```python
from build123d import *

# Parameters (mm, degrees)
SKETCH1_W               = 60
SKETCH1_H               = 30
BOSS_EXTRUDE1_DEPTH     = 3
FILLET2_R               = 2
SKETCH4_W               = 5
SKETCH4_H               = 20
BOSS_EXTRUDE2_DEPTH     = 25
FILLET3_R               = 10
CUT_EXTRUDE3_DEPTH      = 50.145193051
CUT_EXTRUDE3_DEPTH_BACK = 50.145193051
SKETCH5_R               = 2.75
CUT_EXTRUDE4_DEPTH      = 2.5
CHAMFER1_SIZE           = 5


with BuildPart() as part:
    # Sketch1 → Boss-Extrude1 (new body)
    with BuildSketch(Plane(origin=(0, 0, 0), x_dir=(1, 0, 0), z_dir=(0, 1, 0))):
        Rectangle(SKETCH1_W, SKETCH1_H)
    extrude(amount=BOSS_EXTRUDE1_DEPTH)

    # Fillet2
    fillet2_edges = [part.edges().sort_by_distance(p)[0] for p in [
        (-30, 1.5, -15),
        (30, 1.5, -15),
        (30, 1.5, 15),
        (-30, 1.5, 15),
    ]]
    fillet(fillet2_edges, radius=FILLET2_R)

    # Sketch4 → Boss-Extrude2 (add)
    with BuildSketch(Plane(origin=(0, 3, 0), x_dir=(1, 0, 0), z_dir=(0, 1, 0))):
        with Locations((-5, 0)):
            Rectangle(SKETCH4_W, SKETCH4_H)
        with Locations((5, 0)):
            Rectangle(SKETCH4_W, SKETCH4_H)
    extrude(amount=BOSS_EXTRUDE2_DEPTH)

    # Fillet3
    fillet3_edges = [part.edges().sort_by_distance(p)[0] for p in [
        (5, 28, 10),
        (5, 28, -10),
        (-5, 28, -10),
        (-5, 28, 10),
    ]]
    fillet(fillet3_edges, radius=FILLET3_R - 0.0001)  # a hair under: the kernel refuses the full size

    # Sketch5 → Cut-Extrude3 (cut, two sides: drawn at the far end of the back side and taken through both)
    with BuildSketch(Plane.ZY.offset(7.5).offset(-CUT_EXTRUDE3_DEPTH_BACK)):
        with Locations((0, 18)):
            Circle(SKETCH5_R)
    extrude(amount=CUT_EXTRUDE3_DEPTH + CUT_EXTRUDE3_DEPTH_BACK, mode=Mode.SUBTRACT)

    # Sketch6 → Cut-Extrude4 (cut)
    with BuildSketch(Plane(origin=(7.5, 0, 0), x_dir=(0, 0, -1), z_dir=(1, 0, 0))):
        Polygon((0, 13.236860279), (4.125, 15.61843014), (4.125, 20.38156986), (0, 22.763139721), (-4.125, 20.38156986), (-4.125, 15.61843014), align=None)
    extrude(amount=-CUT_EXTRUDE4_DEPTH, mode=Mode.SUBTRACT)

    # Chamfer1
    chamfer1_edges = [part.edges().sort_by_distance(p)[0] for p in [
        (-5, 3, -10),
        (-5, 3, 10),
        (5, 3, -10),
        (5, 3, 10),
    ]]
    chamfer(chamfer1_edges, length=CHAMFER1_SIZE - 0.0001)  # a hair under: the kernel refuses the full size


solid = part.part
```
Design review of the part built by this model. Coordinates are the model's own, in mm. A direction names the side the tool comes from. Round coordinates to 2 decimals unless told otherwise and drop trailing zeros. Write each loop counter-clockwise with the first axis right and the second up, starting at its lowest first coordinate (ties: lowest second). Pieces come first, ordered by that corner, then holes.
Item 1: For faces 4 (the flat face through (0, 3, 0)), 5 (the flat face through (5, 13, -10)), 6 (the flat face through (6.27, 21.59, 2.03)), 7 (the flat face through (-5, 13, 10)), list the 3-axis set-ups (+Z, -Z, +X, -X, +Y, -Y) from which the entire face can be reached by the end or side of a thin tool; tool diameter is ignored.
Item 2: We need section B-B on y = 10. Write out the cut boundary in (x, z), and give its area (3 significant figures).
Item 3: The part is to be moulded in two halves that separate along Y. For faces 1 (the flat face through (7.5, 13, 0)), 2 (the flat face through (5, 6, 12)), 3 (the flat face through (6.268, 14.444, 2.091)), say which applies: +Y half, -Y half, draft (parallel to the pull), parting line (faces both ways), or undercut.
Item 4: We need section C-C on z = -2. Write out the cut boundary in (x, y).
Item 5: Clearance check with flat-ended pins moving along their axes: pin 1 Ø1.5 at (y, z) = (4, 0.5) entering from +X; pin 2 Ø10 at (y, z) = (21.5, -1) entering from -X; pin 3 Ø4 at (x, y) = (4.5, 11) entering from -Z. State where each tip first meets the part, or that it passes through.
Item 6: We need section D-D on z = 3.5. Write out the cut boundary in (x, y), and give its area (3 significant figures).
Item 7: For probe 1 along X at (y, z) = (19, -3.25); probe 2 along Z at (x, y) = (-4.15, 18); probe 3 along Y at (x, z) = (4.35, 0), list the stretches that pass through material, from the lowest coordinate up.
Returned:
1. face 4: +Z, -Z, +Y
1. face 5: -Z, +X, -X, +Y
1. face 6: +X
1. face 7: +Z, +X, -X, +Y
2. outline: (-7.5, -10) - (-2.5, -10) - (-2.5, 10) - (-7.5, 10) - close; (2.5, -10) - (7.5, -10) - (7.5, 10) - (2.5, 10) - close
2. area: 200 mm2
3. face 1: draft
3. face 2: +Y half
3. face 3: undercut
4. outline: (-30, 0) - (30, 0) - (30, 3) - (7.5, 3) - (7.5, 14.39) - (5, 14.39) - (5, 16.11) - (2.5, 16.11) - (2.5, 3) - (-2.5, 3) - (-2.5, 16.11) - (-7.5, 16.11) - (-7.5, 3) - (-30, 3) - close; (-7.5, 19.89) - (-2.5, 19.89) - (-2.5, 27.8) - (-7.5, 27.8) - close; (2.5, 19.89) - (5, 19.89) - (5, 21.61) - (7.5, 21.61) - (7.5, 27.8) - (2.5, 27.8) - close
5. pin 1: stops at x = 7.5
5. pin 2: stops at x = -7.5
5. pin 3: stops at z = -10
6. outline: (-30, 0) - (30, 0) - (30, 3) - (7.5, 3) - (7.5, 15.26) - (5, 15.26) - (5, 20.74) - (7.5, 20.74) - (7.5, 27.37) - (2.5, 27.37) - (2.5, 3) - (-2.5, 3) - (-2.5, 27.37) - (-7.5, 27.37) - (-7.5, 3) - (-30, 3) - close
6. area: 410 mm2
7. probe 1: x = -7.5 to -2.5, 2.5 to 5
7. probe 2: z = -10 to -2.75, 2.75 to 10
7. probe 3: y = 0 to 15.25, 20.75 to 28
